from build123d import *

# Parameters (mm, degrees)
SKETCH_1_W                    = 10
SKETCH_1_H                    = 5
EXTRUDE_1_DEPTH               = 20
M3X0_51_AT_2_COUNT            = 2
M3X0_51_AT_2_PITCH            = 11.5
HOLE_WIZARD_2_561_D           = 1.778
HOLE_WIZARD_2_561_DEPTH       = 5.5
HOLE_WIZARD_2_561_CSINK_D     = 2.54
HOLE_WIZARD_2_561_CSINK_ANGLE = 110
HOLE_WIZARD_2_561_TIP         = 0.53416509


with BuildPart() as part:
    # Эскиз1 → Бобышка-Вытянуть1 (new body)
    with BuildSketch(Plane.XY):
        with Locations((5, 2.5)):
            Rectangle(SKETCH_1_W, SKETCH_1_H)
    extrude(amount=EXTRUDE_1_DEPTH)

    # Эскиз4 → Отверстие обработанное метчиком M3x0.51 (revolve, cut)
    with BuildSketch(Plane(origin=(5, 0, 15), x_dir=(0, 0, -1), z_dir=(1, 0, 0))):
        Polygon((0, 0), (0, 5), (1.65, 5), (1.25, 4.719916985), (1.25, 0.280083015), (1.65, 0), align=None)
    m3x0_51 = revolve(axis=Axis((5, -6.35, 15), (0, 1, 0)), mode=Mode.SUBTRACT)

    # Отверстие обработанное метчиком M3x0.51 at 2: Отверстие обработанное метчиком M3x0.51 ×2
    with Locations(*[(0, 0, -i * M3X0_51_AT_2_PITCH) for i in range(1, M3X0_51_AT_2_COUNT)]):
        add(m3x0_51, mode=Mode.SUBTRACT)

    # Отверстие обработанное метчиком #2-561
    with Locations(Plane.ZY):
        with Locations((3.5, 2.5), (12, 2.5)):
            CounterSinkHole(HOLE_WIZARD_2_561_D / 2, HOLE_WIZARD_2_561_CSINK_D / 2, depth=HOLE_WIZARD_2_561_DEPTH, counter_sink_angle=HOLE_WIZARD_2_561_CSINK_ANGLE)
            with Locations((0, 0, -(HOLE_WIZARD_2_561_DEPTH + HOLE_WIZARD_2_561_TIP / 2))):  # 118° drill point
                Cone(0, HOLE_WIZARD_2_561_D / 2, HOLE_WIZARD_2_561_TIP, mode=Mode.SUBTRACT)


solid = part.part
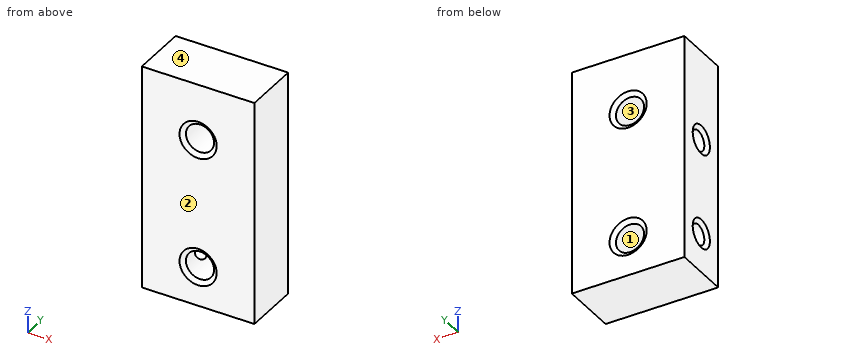
CAD build for the part. Positions are in the model's coordinates, mm. Face numbers are marked on the shaded views. Round coordinates to 2 decimals unless told otherwise and drop trailing zeros. Loops run counter-clockwise (first coordinate to the right, second up) from the corner with the lowest first, then second, coordinate; pieces in that order, holes last. Notation, with made-up numbers: M 60.25,13 L 89.25,13 A25 cw 89.25,25 Z; hole C -4.5,80.25 d2. An arc over 180 degrees is marked long. One line per question, with ' | ' between items. Start each with the question number.
Item 1: Cut at B-B, the plane z = 3.5. Write the cut outline in (x, y).
Item 2: Pin check, flat tip, straight feed: pin 1 Ø2 at (y, z) = (3, 9) entering from -X. Stop position of the tip, or through.
Item 3: Cut at A-A, the plane x = 5. Write the cut outline in (y, z).
Item 4: Cut at D-D, the plane z = 15. Write the cut outline in (x, y), plus the area to 3 significant figures.
Item 5: Two-plate mould, pull along Z, no slides. Class the marked faces 1, 2, 3 and 4: pulls with the +Z half, pulls with the -Z half, needs draft (parallel to the pull), parting line crosses it, or undercut.
Item 6: Cut at C-C, the plane x = 2.75. Write the cut outline in (y, z), plus the area to 3 significant figures.
Item 7: Wall check: line 1 (Z direction, x = 2.35, y = 2.5); line 2 (Y direction, x = 3.3, z = 3.5); line 3 (Z direction, x = 2, y = 2.8). Give the ranges that are in metal, low to high.
Responses:
1) outline: M 0,0 L 3.35,0 L 3.75,0.28 L 3.75,1.61 L 0.27,1.61 L 0,1.23 Z; M 0,3.77 L 0.27,3.39 L 3.75,3.39 L 3.75,4.72 L 3.35,5 L 0,5 Z; M 6.25,0.28 L 6.65,0 L 10,0 L 10,5 L 6.65,5 L 6.25,4.72 Z
2) pin 1: stops at x = 0
3) outline: M 0,0 L 5,0 L 5,1.85 L 4.72,2.25 L 0.28,2.25 L 0,1.85 Z; M 0,5.15 L 0.28,4.75 L 4.72,4.75 L 5,5.15 L 5,13.35 L 4.72,13.75 L 0.28,13.75 L 0,13.35 Z; M 0,16.65 L 0.28,16.25 L 4.72,16.25 L 5,16.65 L 5,20 L 0,20 Z; hole C 2.5,12 d1.78
4) outline: M 0,0 L 3.35,0 L 3.75,0.28 L 3.75,4.72 L 3.35,5 L 0,5 Z; M 6.25,0.28 L 6.65,0 L 10,0 L 10,5 L 6.65,5 L 6.25,4.72 Z | area: 37.3 mm²
5) face 1: undercut | face 2: needs draft | face 3: undercut | face 4: pulls with the +Z half
6) outline: M 0,0 L 5,0 L 5,20 L 0,20 Z; hole C 2.5,3.5 d1.78; hole C 2.5,12 d1.78 | area: 95.0 mm²
7) line 1: z = 0 to 2.61, 4.39 to 11.11, 12.89 to 20 | line 2: y = 0 to 1.61, 3.39 to 5 | line 3: z = 0 to 2.66, 4.34 to 11.16, 12.84 to 20
